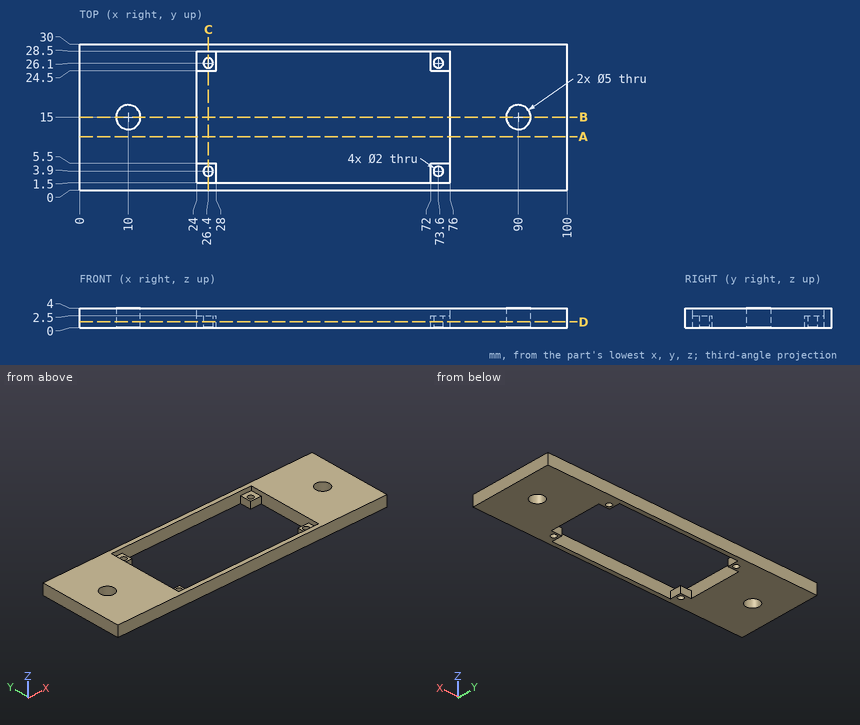
Here's the drawing with two shaded views (mm, measured from the low corner). I have some questions. Coordinates: 2 decimals unless noted, no trailing zeros. Order: outer loops, then holes, each group sorted by start corner. A loop starts at its lowest first (then second) coordinate and runs counter-clockwise, first axis right, second up. Notation, with made-up numbers: (27.25, 30.25) - (48.25, 30.25) arc R21 ccw to (48.25, 69.25) - close; hole circle Ø6 at (-9.75, -9.75). An arc over 180 degrees is marked (long way). Answer in a Markdown table with one row per item. Add a question column.
(1) If we section it at D-D, the plane z = 1.2: Please give me the cut outline in (x, y), then the cut area to 3 significant figures.
(2) If we section it at C-C, the plane x = 26.4: Please give me the cut outline in (y, z), then the cut area to 3 significant figures.
(3) Will these pins go through, and if not, where does the flat tip stop? pin 1 (2 mm diameter, centred on x = 74.5, y = 4.5, fed in from +Z); pin 2 (1.2 mm diameter, centred on x = 59, z = 1.5, fed in from -Y).
(4) If we section it at B-B, the plane y = 15: Please give me the cut outline in (x, z).
(5) I need wall thicknesses on L1, parallel to X at y = 4, z = 1.1; L2, parallel to Y at x = 26.4, z = 0.85; L3, parallel to Y at x = 73.5, z = 3.6. Which ranges of each line are inside material? Lowest first, please.
(6) If we section it at A-A, the plane y = 11: Please give me the cut outline in (x, z).
Results are:
| question | item | result |
|---|---|---|
| 1 | outline | (0, 0) - (100, 0) - (100, 30) - (0, 30) - close; hole circle Ø5 at (10, 15); hole (24, 5.5) - (28, 5.5) - (28, 1.5) - (72, 1.5) - (72, 5.5) - (76, 5.5) - (76, 24.5) - (72, 24.5) - (72, 28.5) - (28, 28.5) - (28, 24.5) - (24, 24.5) - close; hole circle Ø2 at (26.4, 3.9); hole circle Ø2 at (26.4, 26.1); hole circle Ø2 at (73.6, 3.9); hole circle Ø2 at (73.6, 26.1); hole circle Ø5 at (90, 15) |
| 1 | area | 1,610 mm2 |
| 2 | outline | (0, 0) - (2.9, 0) - (2.9, 2.5) - (1.5, 2.5) - (1.5, 4) - (0, 4) - close; (4.9, 0) - (5.5, 0) - (5.5, 2.5) - (4.9, 2.5) - close; (24.5, 0) - (25.1, 0) - (25.1, 2.5) - (24.5, 2.5) - close; (27.1, 0) - (30, 0) - (30, 4) - (28.5, 4) - (28.5, 2.5) - (27.1, 2.5) - close |
| 2 | area | 22.0 mm2 |
| 3 | pin 1 | stops at z = 2.5 |
| 3 | pin 2 | stops at y = 0 |
| 4 | outline | (0, 0) - (7.5, 0) - (7.5, 4) - (0, 4) - close; (12.5, 0) - (24, 0) - (24, 4) - (12.5, 4) - close; (76, 0) - (87.5, 0) - (87.5, 4) - (76, 4) - close; (92.5, 0) - (100, 0) - (100, 4) - (92.5, 4) - close |
| 5 | L1 | x = 0 to 25.41, 27.39 to 28, 72 to 72.61, 74.59 to 100 |
| 5 | L2 | y = 0 to 2.9, 4.9 to 5.5, 24.5 to 25.1, 27.1 to 30 |
| 5 | L3 | y = 0 to 1.5, 28.5 to 30 |
| 6 | outline | (0, 0) - (24, 0) - (24, 4) - (0, 4) - close; (76, 0) - (100, 0) - (100, 4) - (76, 4) - close |
